The figure shows three views and two pictorial views of one solid part (mm, origin at its lowest corner). Answer the questions. A direction names the side the tool comes from. Round coordinates to 2 decimals unless told otherwise and drop trailing zeros. Write each loop counter-clockwise with the first axis right and the second up, starting at its lowest first coordinate (ties: lowest second). Pieces come first, ordered by that corner, then holes.
Item 1: A tool of negligible diameter and unlimited length cuts with its end or side. For the marked faces 1, 2 and 3, from which of +Z, -Z, +X, -X, +Y, -Y can it reach the whole face along a straight path? Write none if from no direction.
Item 2: Find section C-C on y = 3. Give the vertices of the cut face in (x, z), then the cut area to 3 significant figures.
Item 3: This flat-tipped pin is pushed along its axis until it touches: pin 1 (1 mm diameter, centred on x = 1, z = 1.5, fed in from -Y). Where does it stop, or does it pass through?
Item 4: Find section B-B on z = 1.1. Give the vertices of the cut face in (x, y), then the cut area to 3 significant figures.
Item 5: Find section D-D on x = 7.25. Give the vertices of the cut face in (y, z).
Item 6: Find section A-A on y = 2.1. Give the vertices of the cut face in (x, z), then the cut area to 3 significant figures.
Item 7: Find the intervals of material crossed by probe 1 along Y at (x, z) = (0.75, 0.9); probe 2 along X at (y, z) = (4.1, 1.75); probe 3 along X at (y, z) = (4.2, 1.6), in increasing order.
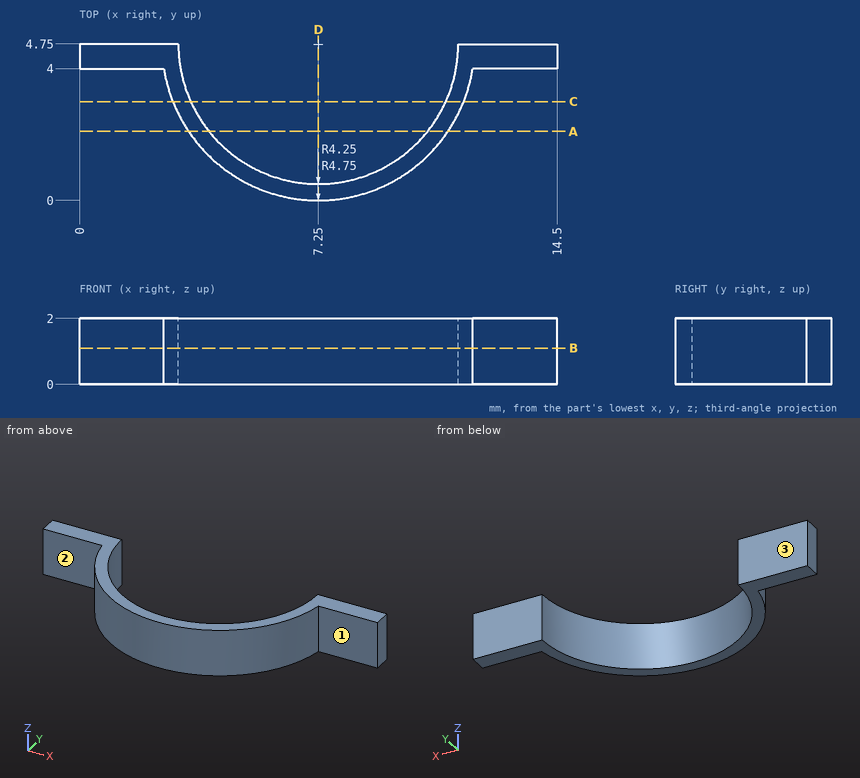
Check values:
1. face 1: +Z, -Z, +X, -Y
1. face 2: +Z, -Z, -X, -Y
1. face 3: +Z, -Z, +X, -X, +Y
2. outline: (2.83, 0) - (3.38, 0) - (3.38, 2) - (2.83, 2) - close; (11.12, 0) - (11.67, 0) - (11.67, 2) - (11.12, 2) - close
2. area: 2.17 mm2
3. pin 1: stops at y = 4
4. outline: (0, 4) - (2.56, 4) arc R4.75 ccw to (11.94, 4) - (14.5, 4) - (14.5, 4.75) - (11.5, 4.75) arc R4.25 cw to (3, 4.75) - (0, 4.75) - close
4. area: 10.8 mm2
5. outline: (0, 0) - (0.5, 0) - (0.5, 2) - (0, 2) - close
6. outline: (3.31, 0) - (3.93, 0) - (3.93, 2) - (3.31, 2) - close; (10.57, 0) - (11.19, 0) - (11.19, 2) - (10.57, 2) - close
6. area: 2.48 mm2
7. probe 1: y = 4 to 4.75
7. probe 2: x = 0 to 3.05, 11.45 to 14.5
7. probe 3: x = 0 to 3.04, 11.46 to 14.5
